Here's how the part is built. I have some questions about the finished solid (model axes, mm). A direction names the side the tool comes from. Give positions to 0.01 mm unless a question says otherwise; leave off trailing zeros. Write each loop counter-clockwise with the first axis right and the second up, starting at its lowest first coordinate (ties: lowest second). Pieces come first, ordered by that corner, then holes. Notation, with made-up numbers: (89.5, 15) -> (133.5, 15) arc R18 cw to (133.5, 21) -> close; hole circle Ø3 at (81.25, 6.5). An arc over 180 degrees is marked (long way). Return JSON: item names as keys, results as strings.
from build123d import *

# Parameters (mm, degrees)
SKETCH1_W                     = 79
SKETCH1_H                     = 40
BOSS_EXTRUDE1_DEPTH           = 3.175
SKETCH2_W                     = 3.175
SKETCH2_H                     = 6.35
CUT_EXTRUDE1_DEPTH            = 10
LPATTERN1_COUNT               = 6
LPATTERN1_PITCH               = 6.35
LPATTERN1_COPY_1_SKETCH_W     = 3.175
LPATTERN1_COPY_1_SKETCH_H     = 6.35
LPATTERN1_COPY_1_DEPTH        = 10
LPATTERN1_COPY_2_SKETCH_W     = 3.175
LPATTERN1_COPY_2_SKETCH_H     = 6.35
LPATTERN1_COPY_2_DEPTH        = 10
LPATTERN1_COPY_3_SKETCH_W     = 3.175
LPATTERN1_COPY_3_SKETCH_H     = 6.35
LPATTERN1_COPY_3_DEPTH        = 10
LPATTERN1_COPY_4_SKETCH_W     = 3.175
LPATTERN1_COPY_4_SKETCH_H     = 6.35
LPATTERN1_COPY_4_DEPTH        = 10
LPATTERN1_COPY_5_SKETCH_W     = 3.175
LPATTERN1_COPY_5_SKETCH_H     = 6.35
LPATTERN1_COPY_5_DEPTH        = 10
LPATTERN1_COL_COUNT           = 6
LPATTERN1_COL_PITCH           = 6.35
LPATTERN1_COL_COPY_1_SKETCH_W = 3.175
LPATTERN1_COL_COPY_1_SKETCH_H = 6.35
LPATTERN1_COL_COPY_1_DEPTH    = 10
LPATTERN1_COL_COPY_2_SKETCH_W = 3.175
LPATTERN1_COL_COPY_2_SKETCH_H = 6.35
LPATTERN1_COL_COPY_2_DEPTH    = 10
LPATTERN1_COL_COPY_3_SKETCH_W = 3.175
LPATTERN1_COL_COPY_3_SKETCH_H = 6.35
LPATTERN1_COL_COPY_3_DEPTH    = 10
LPATTERN1_COL_COPY_4_SKETCH_W = 3.175
LPATTERN1_COL_COPY_4_SKETCH_H = 6.35
LPATTERN1_COL_COPY_4_DEPTH    = 10
LPATTERN1_COL_COPY_5_SKETCH_W = 3.175
LPATTERN1_COL_COPY_5_SKETCH_H = 6.35
LPATTERN1_COL_COPY_5_DEPTH    = 10
SKETCH3_W                     = 6.35
SKETCH3_H                     = 3.175
BOSS_EXTRUDE2_DEPTH           = 3.175
LPATTERN2_COUNT               = 3
LPATTERN2_PITCH               = 6.35
LPATTERN2_COL_COUNT           = 3
LPATTERN2_COL_PITCH           = 6.35
MIRROR2_COPY_1_SKETCH_W       = 6.35
MIRROR2_COPY_1_SKETCH_H       = 3.175
MIRROR2_COPY_1_DEPTH          = 3.175
MIRROR2_COPY_2_SKETCH_W       = 6.35
MIRROR2_COPY_2_SKETCH_H       = 3.175
MIRROR2_COPY_2_DEPTH          = 3.175
MIRROR2_COPY_3_SKETCH_W       = 6.35
MIRROR2_COPY_3_SKETCH_H       = 3.175
MIRROR2_COPY_3_DEPTH          = 3.175
MIRROR2_COPY_4_SKETCH_W       = 6.35
MIRROR2_COPY_4_SKETCH_H       = 3.175
MIRROR2_COPY_4_DEPTH          = 3.175


with BuildPart() as part:
    # Sketch1 → Boss-Extrude1 (new body)
    with BuildSketch(Plane.XY):
        Rectangle(SKETCH1_W, SKETCH1_H)
    extrude(amount=BOSS_EXTRUDE1_DEPTH)

    # Sketch2 → Cut-Extrude1 (cut)
    with BuildSketch(Plane.XY.offset(3.175)):
        with Locations((0, -20)):
            Rectangle(SKETCH2_W, SKETCH2_H)
    cut_extrude1 = extrude(amount=-CUT_EXTRUDE1_DEPTH, mode=Mode.SUBTRACT)

    # Mirror1: Cut-Extrude1 across plane
    add(cut_extrude1.mirror(Plane.ZX), mode=Mode.SUBTRACT)

    # LPattern1: Cut-Extrude1 ×6
    with Locations(*[(i * LPATTERN1_PITCH, 0, 0) for i in range(1, LPATTERN1_COUNT)]):
        add(cut_extrude1, mode=Mode.SUBTRACT)

    # LPattern1 copy 1 sketch → LPattern1 copy 1 (cut)
    with BuildSketch(Plane(origin=(6.35, 0, 3.175), x_dir=(1, 0, 0), z_dir=(0, 0, 1))):
        with Locations((0, 20)):
            Rectangle(LPATTERN1_COPY_1_SKETCH_W, LPATTERN1_COPY_1_SKETCH_H)
    extrude(amount=-LPATTERN1_COPY_1_DEPTH, mode=Mode.SUBTRACT)

    # LPattern1 copy 2 sketch → LPattern1 copy 2 (cut)
    with BuildSketch(Plane(origin=(12.7, 0, 3.175), x_dir=(1, 0, 0), z_dir=(0, 0, 1))):
        with Locations((0, 20)):
            Rectangle(LPATTERN1_COPY_2_SKETCH_W, LPATTERN1_COPY_2_SKETCH_H)
    extrude(amount=-LPATTERN1_COPY_2_DEPTH, mode=Mode.SUBTRACT)

    # LPattern1 copy 3 sketch → LPattern1 copy 3 (cut)
    with BuildSketch(Plane(origin=(19.05, 0, 3.175), x_dir=(1, 0, 0), z_dir=(0, 0, 1))):
        with Locations((0, 20)):
            Rectangle(LPATTERN1_COPY_3_SKETCH_W, LPATTERN1_COPY_3_SKETCH_H)
    extrude(amount=-LPATTERN1_COPY_3_DEPTH, mode=Mode.SUBTRACT)

    # LPattern1 copy 4 sketch → LPattern1 copy 4 (cut)
    with BuildSketch(Plane(origin=(25.4, 0, 3.175), x_dir=(1, 0, 0), z_dir=(0, 0, 1))):
        with Locations((0, 20)):
            Rectangle(LPATTERN1_COPY_4_SKETCH_W, LPATTERN1_COPY_4_SKETCH_H)
    extrude(amount=-LPATTERN1_COPY_4_DEPTH, mode=Mode.SUBTRACT)

    # LPattern1 copy 5 sketch → LPattern1 copy 5 (cut)
    with BuildSketch(Plane(origin=(31.75, 0, 3.175), x_dir=(1, 0, 0), z_dir=(0, 0, 1))):
        with Locations((0, 20)):
            Rectangle(LPATTERN1_COPY_5_SKETCH_W, LPATTERN1_COPY_5_SKETCH_H)
    extrude(amount=-LPATTERN1_COPY_5_DEPTH, mode=Mode.SUBTRACT)

    # LPattern1 col: Cut-Extrude1 ×6
    with Locations(*[(-i * LPATTERN1_COL_PITCH, 0, 0) for i in range(1, LPATTERN1_COL_COUNT)]):
        add(cut_extrude1, mode=Mode.SUBTRACT)

    # LPattern1 col copy 1 sketch → LPattern1 col copy 1 (cut)
    with BuildSketch(Plane(origin=(-6.35, 0, 3.175), x_dir=(1, 0, 0), z_dir=(0, 0, 1))):
        with Locations((0, 20)):
            Rectangle(LPATTERN1_COL_COPY_1_SKETCH_W, LPATTERN1_COL_COPY_1_SKETCH_H)
    extrude(amount=-LPATTERN1_COL_COPY_1_DEPTH, mode=Mode.SUBTRACT)

    # LPattern1 col copy 2 sketch → LPattern1 col copy 2 (cut)
    with BuildSketch(Plane(origin=(-12.7, 0, 3.175), x_dir=(1, 0, 0), z_dir=(0, 0, 1))):
        with Locations((0, 20)):
            Rectangle(LPATTERN1_COL_COPY_2_SKETCH_W, LPATTERN1_COL_COPY_2_SKETCH_H)
    extrude(amount=-LPATTERN1_COL_COPY_2_DEPTH, mode=Mode.SUBTRACT)

    # LPattern1 col copy 3 sketch → LPattern1 col copy 3 (cut)
    with BuildSketch(Plane(origin=(-19.05, 0, 3.175), x_dir=(1, 0, 0), z_dir=(0, 0, 1))):
        with Locations((0, 20)):
            Rectangle(LPATTERN1_COL_COPY_3_SKETCH_W, LPATTERN1_COL_COPY_3_SKETCH_H)
    extrude(amount=-LPATTERN1_COL_COPY_3_DEPTH, mode=Mode.SUBTRACT)

    # LPattern1 col copy 4 sketch → LPattern1 col copy 4 (cut)
    with BuildSketch(Plane(origin=(-25.4, 0, 3.175), x_dir=(1, 0, 0), z_dir=(0, 0, 1))):
        with Locations((0, 20)):
            Rectangle(LPATTERN1_COL_COPY_4_SKETCH_W, LPATTERN1_COL_COPY_4_SKETCH_H)
    extrude(amount=-LPATTERN1_COL_COPY_4_DEPTH, mode=Mode.SUBTRACT)

    # LPattern1 col copy 5 sketch → LPattern1 col copy 5 (cut)
    with BuildSketch(Plane(origin=(-31.75, 0, 3.175), x_dir=(1, 0, 0), z_dir=(0, 0, 1))):
        with Locations((0, 20)):
            Rectangle(LPATTERN1_COL_COPY_5_SKETCH_W, LPATTERN1_COL_COPY_5_SKETCH_H)
    extrude(amount=-LPATTERN1_COL_COPY_5_DEPTH, mode=Mode.SUBTRACT)

    # Sketch3 → Boss-Extrude2 (add)
    with BuildSketch(Plane.XY.offset(3.175)):
        with Locations((-39.5, 0)):
            Rectangle(SKETCH3_W, SKETCH3_H)
    boss_extrude2 = extrude(amount=-BOSS_EXTRUDE2_DEPTH)

    # LPattern2: Boss-Extrude2 ×3
    with Locations(*[(0, i * LPATTERN2_PITCH, 0) for i in range(1, LPATTERN2_COUNT)]):
        add(boss_extrude2)

    # LPattern2 col: Boss-Extrude2 ×3
    with Locations(*[(0, -i * LPATTERN2_COL_PITCH, 0) for i in range(1, LPATTERN2_COL_COUNT)]):
        add(boss_extrude2)

    # Mirror2: Boss-Extrude2 across plane
    add(boss_extrude2.mirror(Plane(origin=(0, 0, 0), x_dir=(0, 0, 1), z_dir=(1, 0, 0))))

    # Mirror2 copy 1 sketch → Mirror2 copy 1 (add)
    with BuildSketch(Plane(origin=(0, 6.35, 3.175), x_dir=(-1, 0, 0), z_dir=(0, 0, 1))):
        with Locations((-39.5, 0)):
            Rectangle(MIRROR2_COPY_1_SKETCH_W, MIRROR2_COPY_1_SKETCH_H)
    extrude(amount=-MIRROR2_COPY_1_DEPTH)

    # Mirror2 copy 2 sketch → Mirror2 copy 2 (add)
    with BuildSketch(Plane(origin=(0, 12.7, 3.175), x_dir=(-1, 0, 0), z_dir=(0, 0, 1))):
        with Locations((-39.5, 0)):
            Rectangle(MIRROR2_COPY_2_SKETCH_W, MIRROR2_COPY_2_SKETCH_H)
    extrude(amount=-MIRROR2_COPY_2_DEPTH)

    # Mirror2 copy 3 sketch → Mirror2 copy 3 (add)
    with BuildSketch(Plane(origin=(0, -6.35, 3.175), x_dir=(-1, 0, 0), z_dir=(0, 0, 1))):
        with Locations((-39.5, 0)):
            Rectangle(MIRROR2_COPY_3_SKETCH_W, MIRROR2_COPY_3_SKETCH_H)
    extrude(amount=-MIRROR2_COPY_3_DEPTH)

    # Mirror2 copy 4 sketch → Mirror2 copy 4 (add)
    with BuildSketch(Plane(origin=(0, -12.7, 3.175), x_dir=(-1, 0, 0), z_dir=(0, 0, 1))):
        with Locations((-39.5, 0)):
            Rectangle(MIRROR2_COPY_4_SKETCH_W, MIRROR2_COPY_4_SKETCH_H)
    extrude(amount=-MIRROR2_COPY_4_DEPTH)


solid = part.part
1. Suppose I cut it at A-A, the plane y = 2.5. List the corners of the cut face in (x, z) for me (3 decimals), and give its area (3 significant figures).
Taken from the geometry:
{"outline": "(-39.5, 0) -> (39.5, 0) -> (39.5, 3.175) -> (-39.5, 3.175) -> close", "area": "251 mm²"}
2. If I drill on line 1 (Y direction, x = -20, z = 1.2) (3 decimals); line 2 (X direction, y = 11, z = 1.8), over which ranges is the centre line in solid material (lowest first)? Write a range as [from, to].
Taken from the geometry:
{"line 1": "y = [-16.825, 16.825]", "line 2": "x = [-39.5, 39.5]"}
3. Which directions (+Z, -Z, +X, -X, +Y, -Y) give clear straight access to the entire face, cutting with the end or side of a thin tool? Please do faces 4 (the face through (-39.5, -3, 2)), 5 (the face through (41, 7.938, 2)), 6 (the face through (7.938, -18, 2)), 7 (the face through (29, -20, 2)), 8 (the face through (19, 16.825, 2)).
Taken from the geometry:
{"face 4": "+Z, -Z, -X", "face 5": "+Z, -Z, +X", "face 6": "+Z, -Z, -Y", "face 7": "+Z, -Z, +X, -X, -Y", "face 8": "+Z, -Z, +Y"}
4. If we mould it in two halves opening along X, with no side actions, what happens to faces 1 (the face through (39.5, 3, 2)), 2 (the face through (16, 20, 2)), 3 (the face through (4.762, 18, 2))? For each: released by +X, released by -X, zero draft, split by the parting line, or undercut.
Taken from the geometry:
{"face 1": "released by +X", "face 2": "zero draft", "face 3": "undercut"}
5. For pin 1 Ø1 at (y, z) = (9, 1.5) entering from -X; pin 2 Ø1.6 at (y, z) = (18, 1) entering from +X, each with a flat end and sliding along its axis, tell me the tip position at first contact or that it passes through.
Taken from the geometry:
{"pin 1": "stops at x = -39.5", "pin 2": "stops at x = 39.5"}
